Design review of the part shown in the three views and the two pictorial views. Dimensions are in mm from the part's minimum x, y and z. Coordinates: 2 decimals unless noted, no trailing zeros. Loops run counter-clockwise (first coordinate to the right, second up) from the corner with the lowest first, then second, coordinate; pieces in that order, holes last. Notation, with made-up numbers: M -24.5,74 L 18.5,74 A12 ccw 18.5,81 Z; hole C -8.5,29.25 d11. An arc over 180 degrees is marked long. Answer as a JSON object with one key per item and string values. Group by question number.
Item 1: Add section B-B (z = 12). State the section outline as (x, y) points (1 decimal).
Item 2: Wall thickness on L1, parallel to Z at x = 7, y = 21; L2, parallel to Z at x = 11.5, y = 21; L3, parallel to Y at x = 5.25, z = 14: over which ranges is each line inside the solid? List them lowest first. Write a range as from..to.
Item 3: Add section C-C (x = 11.25). State the section outline as (y, z) points (1 decimal), then the cut area to 3 significant figures.
Item 4: Add section D-D (x = 14.75). State the section outline as (y, z) points (1 decimal).
Item 5: Insertion check: pin 1 (10 mm diameter, centred on x = 3, z = 33.5, fed in from -Y) (1 decimal); pin 2 (4 mm diameter, centred on x = 12.5, y = 36.5, fed in from -Z); pin 3 (12 mm diameter, centred on x = 18, y = 37, fed in from -Z). Each pin has a flat end and moves straight along its axis. Give the tip position at first contact, or say it passes through.
Item 6: Add section A-A (y = 25). State the section outline as (x, z) points (1 decimal).
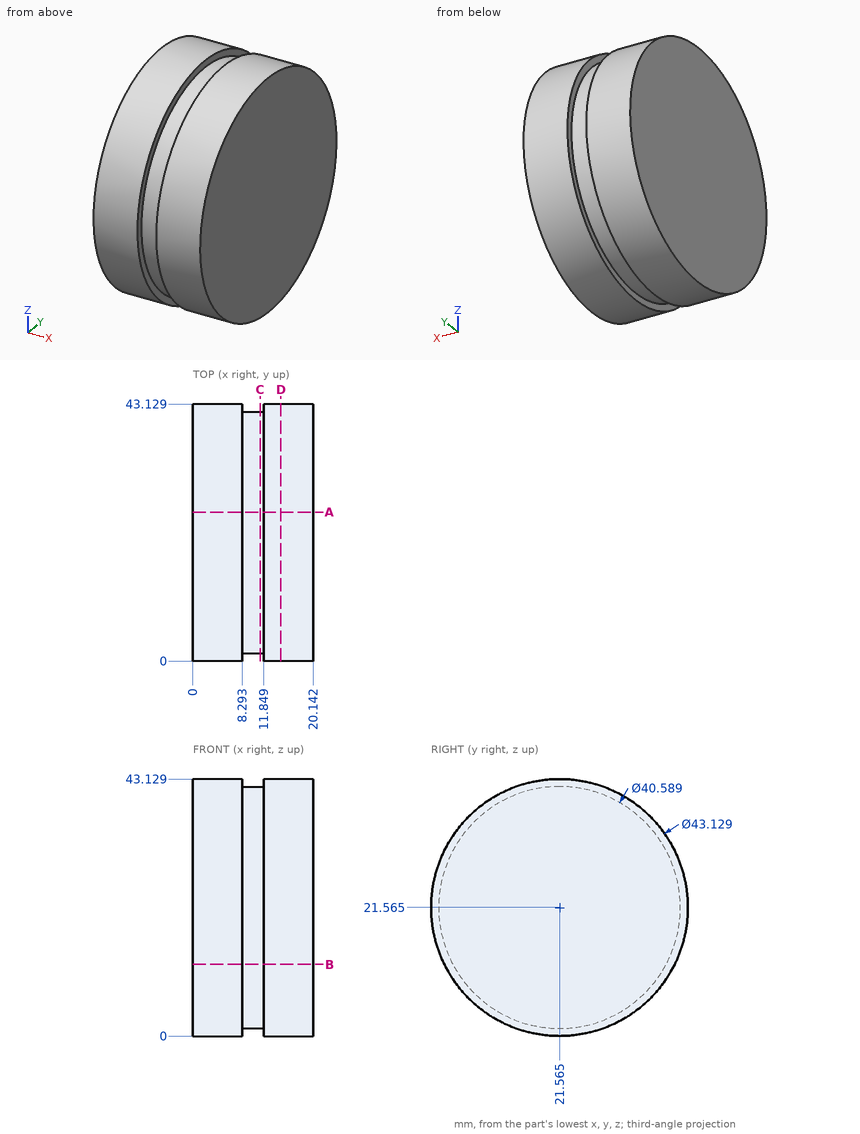
From the geometry:
{
 "1": {"outline": "M 0,2.2 L 8.3,2.2 L 8.3,3.7 L 11.8,3.7 L 11.8,2.2 L 20.1,2.2 L 20.1,40.9 L 11.8,40.9 L 11.8,39.5 L 8.3,39.5 L 8.3,40.9 L 0,40.9 Z"},
 "2": {"L1": "z = 0.01..43.12", "L2": "z = 1.28..41.85", "L3": "y = 1.37..41.76"},
 "3": {"outline": "C 21.6,21.6 d40.6", "area": "1,290 mm²"},
 "4": {"outline": "C 21.6,21.6 d43.1"},
 "5": {"pin 1": "stops at y = 1.1", "pin 2": "stops at z = 4.31", "pin 3": "stops at z = 2.17"},
 "6": {"outline": "M 0,0.3 L 8.3,0.3 L 8.3,1.6 L 11.8,1.6 L 11.8,0.3 L 20.1,0.3 L 20.1,42.9 L 11.8,42.9 L 11.8,41.6 L 8.3,41.6 L 8.3,42.9 L 0,42.9 Z"}
}
